Source: CAD feature listing. Evaluate the final solid. Frame: model axes, mm. Face numbers are marked on the shaded views. Give positions to 0.01 mm unless a question says otherwise; leave off trailing zeros. Order: outer loops, then holes, each group sorted by start corner. A loop starts at its lowest first (then second) coordinate and runs counter-clockwise, first axis right, second up. Notation, with made-up numbers: (9.25, -29.75) - (17.25, -29.75) arc R12 ccw to (17.25, -7.75) - close; hole circle Ø9 at (-2.75, 62). An arc over 180 degrees is marked (long way). One line per item, written item: value. Start each with the question number.
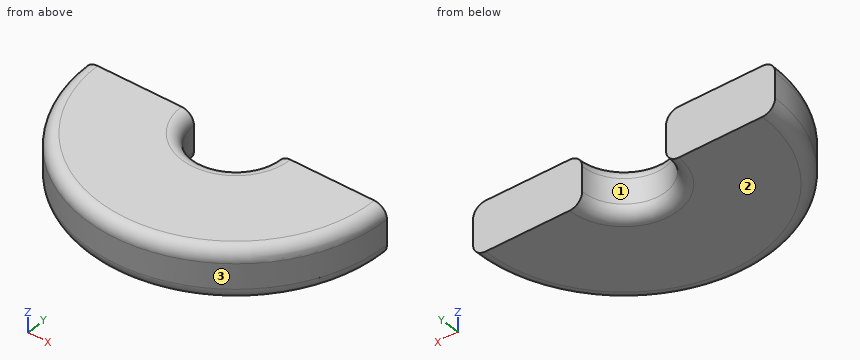
from build123d import *

# Parameters (mm, degrees)
F1_ANGLE = 180


with BuildPart() as f1:
    # F0 (on Front) → F1 (revolve)
    with BuildSketch(Plane.XZ):
        with BuildLine():
            Line((-16.51, 7.62), (-41.91, 7.62))
            ThreePointArc((-41.91, 7.62), (-44.604077, 6.504077), (-45.72, 3.81))
            Line((-45.72, 3.81), (-45.72, -3.81))
            ThreePointArc((-45.72, -3.81), (-44.604077, -6.504077), (-41.91, -7.62))
            Line((-41.91, -7.62), (-16.51, -7.62))
            ThreePointArc((-16.51, -7.62), (-13.815923, -6.504077), (-12.7, -3.81))
            Line((-12.7, -3.81), (-12.7, 3.81))
            ThreePointArc((-12.7, 3.81), (-13.815923, 6.504077), (-16.51, 7.62))
        make_face()
    revolve(axis=Axis((0, 0, 0), (0, 0, 1)), revolution_arc=F1_ANGLE)


solid = f1.part
1. Section A-A on x = 0. Return the cut outline in (y, z), then the cut area to 3 significant figures.
2. Contact query for flat-ended pins moving along their axis: pin 1 Ø6 at (x, y) = (29.5, -40) entering from +Z; pin 2 Ø4 at (y, z) = (-10, -1.5) entering from +X; pin 3 Ø1 at (y, z) = (-18, -4.5) entering from -X; pin 4 Ø6 at (x, z) = (-11.5, -2) entering from -Y. Output: stop coordinate, or through.
3. Section B-B on z = 0.5. Return the cut outline in (x, y), then the cut area to 3 significant figures.
4. Section C-C on z = 6. Return the cut outline in (x, y).
5. Ray query, L1, parallel to Y at x = -20, z = -3; L2, parallel to Y at x = -22.5, z = 7; L3, parallel to X at y = -13.5, z = -3.75. Return the intervals inside material, ascending.
6. Draft query along X for the marked faces 1, 2 and 3. Return one class per face: pulls with the +X half, pulls with the -X half, needs draft (parallel to the pull), parting line crosses it, or undercut.
Data:
1. outline: (-45.72, -3.81) arc R3.81 ccw to (-41.91, -7.62) - (-16.51, -7.62) arc R3.81 ccw to (-12.7, -3.81) - (-12.7, 3.81) arc R3.81 ccw to (-16.51, 7.62) - (-41.91, 7.62) arc R3.81 ccw to (-45.72, 3.81) - close
1. area: 491 mm2
2. pin 1: passes through
2. pin 2: stops at x = 45.01
2. pin 3: stops at x = -42.19
2. pin 4: stops at y = -44.92
3. outline: (-45.72, 0) arc R45.72 ccw to (45.72, 0) - (12.7, 0) arc R12.7 cw to (-12.7, 0) - close
3. area: 3,030 mm2
4. outline: (-45.03, 0) arc R45.03 ccw to (45.03, 0) - (13.39, 0) arc R13.39 cw to (-13.39, 0) - close
5. L1: y = -41.11 to 0
5. L2: y = -37.8 to 0
5. L3: x = -43.68 to 43.68
6. face 1: undercut
6. face 2: needs draft
6. face 3: parting line crosses it
